```python
from build123d import *

# Parameters (mm, degrees)
SKETCH_1_W          = 20
SKETCH_1_H          = 40
EXTRUDE_1_DEPTH     = 32.5
SKETCH_2_W          = 20
SKETCH_2_H          = 55
EXTRUDE_2_DEPTH     = 2.5
SKETCH_3_W          = 20
SKETCH_3_H          = 40
EXTRUDE_3_DEPTH     = 8
SKETCH_4_R          = 3
EXTRUDE_4_DEPTH     = 5
SKETCH_5_R          = 1.5
CUT_EXTRUDE_1_DEPTH = 36


with BuildPart() as part:
    # 草图1 → 凸台-拉伸1 (new body)
    with BuildSketch(Plane.XY):
        Rectangle(SKETCH_1_W, SKETCH_1_H)
    extrude(amount=EXTRUDE_1_DEPTH)

    # 草图2 → 凸台-拉伸2 (add)
    with BuildSketch(Plane.XY.offset(32.5)):
        Rectangle(SKETCH_2_W, SKETCH_2_H)
    extrude(amount=EXTRUDE_2_DEPTH)

    # 草图3 → 凸台-拉伸3 (add)
    with BuildSketch(Plane.XY.offset(35)):
        Rectangle(SKETCH_3_W, SKETCH_3_H)
    extrude(amount=EXTRUDE_3_DEPTH)

    # 草图4 → 凸台-拉伸4 (add)
    with BuildSketch(Plane.XY.offset(43)):
        with Locations((0, 10.35)):
            Circle(SKETCH_4_R)
    extrude(amount=EXTRUDE_4_DEPTH)

    # 草图5 → 切除-拉伸1 (cut, through all)
    with BuildSketch(Plane.XY.offset(35)):
        with Locations((-5, 24.315)):
            Circle(SKETCH_5_R)
        with Locations((5, 24.315)):
            Circle(SKETCH_5_R)
        with Locations((-5, -24.315)):
            Circle(SKETCH_5_R)
        with Locations((5, -24.315)):
            Circle(SKETCH_5_R)
    extrude(amount=-CUT_EXTRUDE_1_DEPTH, mode=Mode.SUBTRACT)


solid = part.part
```
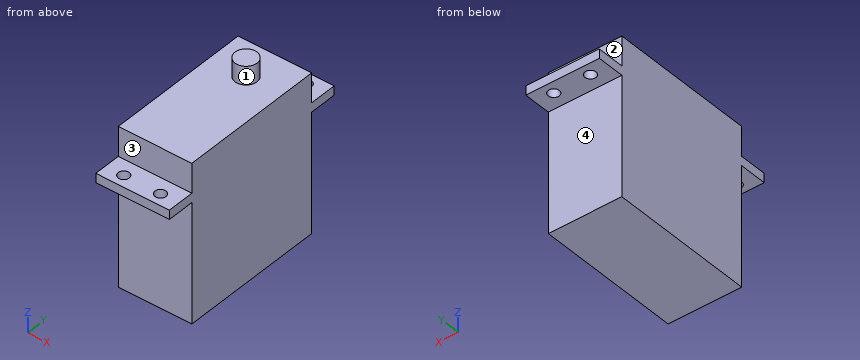
CAD build for the part. Positions are in the model's coordinates, mm. Face numbers are marked on the shaded views. A direction names the side the tool comes from. Give positions to 0.01 mm unless a question says otherwise; leave off trailing zeros. Order: outer loops, then holes, each group sorted by start corner. A loop starts at its lowest first (then second) coordinate and runs counter-clockwise, first axis right, second up. Notation, with made-up numbers: M 42,35.5 L 88,35.5 A17 ccw 88,39.5 Z; hole C 51.25,-16 d11. An arc over 180 degrees is marked long. Put each result on its own line as item: value. Start each with the question number.
(1) Saw through at D-D, the plane z = 23.5. Write the cut outline in (x, y).
(2) Saw through at B-B, the plane y = 10.35. Write the cut outline in (x, z).
(3) Which spindle directions (+Z, -Z, +X, -X, +Y, -Y) get a long thin tool onto all of the face, cutting with end or side? Do the marked faces 1, 2, 3 and 4. Say none if no direction does.
(4) Drill centre lines: line 1 along Y through (x, z) = (-5, 34.4) (3 decimals); line 2 along Y through (x, z) = (-5.5, 36); line 3 along Z through (x, y) = (1, 23). Where is each one in solid material? Low to high.
(5) Flat gauge pins, fed straight in: pin 1 Ø6.5 at (x, z) = (-2, 38) entering from +Y; pin 2 Ø2.5 at (x, y) = (5, 24.315) entering from +Z; pin 3 Ø2 at (x, y) = (-2, -22) entering from -Z; pin 4 Ø2 at (x, z) = (2, 27.5) entering from -Y. Where does each tip first touch, or does it go through?
(6) Saw through at C-C, the plane x = 0. Write the cut outline in (y, z).
(7) Saw through at A-A, the plane x = 5. Write the cut outline in (y, z) (3 decimals).
Check result:
1. outline: M -10,-20 L 10,-20 L 10,20 L -10,20 Z
2. outline: M -10,0 L 10,0 L 10,43 L 3,43 L 3,48 L -3,48 L -3,43 L -10,43 Z
3. face 1: +Z
3. face 2: +Z, +X, -X, +Y
3. face 3: +Z, +X, -X, -Y
3. face 4: -Z, +X, -X, +Y
4. line 1: y = -27.5 to -25.815, -22.815 to 22.815, 25.815 to 27.5
4. line 2: y = -20 to 20
4. line 3: z = 32.5 to 35
5. pin 1: stops at y = 27.5
5. pin 2: passes through
5. pin 3: stops at z = 32.5
5. pin 4: stops at y = -20
6. outline: M -27.5,32.5 L -20,32.5 L -20,0 L 20,0 L 20,32.5 L 27.5,32.5 L 27.5,35 L 20,35 L 20,43 L 13.35,43 L 13.35,48 L 7.35,48 L 7.35,43 L -20,43 L -20,35 L -27.5,35 Z
7. outline: M -27.5,32.5 L -25.815,32.5 L -25.815,35 L -27.5,35 Z; M -22.815,32.5 L -20,32.5 L -20,0 L 20,0 L 20,32.5 L 22.815,32.5 L 22.815,35 L 20,35 L 20,43 L -20,43 L -20,35 L -22.815,35 Z; M 25.815,32.5 L 27.5,32.5 L 27.5,35 L 25.815,35 Z
